```python
from build123d import *

# Parameters (mm, degrees)
F1_DEPTH = 11
F3_DEPTH = 25
F4_W     = 3.629314
F4_H     = 7.762888
F5_DEPTH = 35
F6_R     = 3
F7_DEPTH = 7.75
F8_R     = 1.5
F9_DEPTH = 25


with BuildPart() as f1:
    # F0 (on Top) → F1 (new body)
    with BuildSketch(Plane.XY):
        with BuildLine():
            Line((1.2, 0), (3, 0))
            ThreePointArc((3, 0), (2.12132, 2.12132), (0, 3))
            Line((0, 3), (0, 1.2))
            Line((0, 1.2), (1.2, 1.2))
            Line((1.2, 1.2), (1.2, 1.0315))
            Line((1.2, 1.0315), (1.2, 0.863))
            Line((1.2, 0.863), (1.2, 0))
        make_face()
        with BuildLine():
            ThreePointArc((0, -3), (2.12132, -2.12132), (3, 0))
            Line((3, 0), (1.2, 0))
            Line((1.2, 0), (1.2, -1.2))
            Line((1.2, -1.2), (0, -1.2))
            Line((0, -1.2), (0, -3))
        make_face()
        with BuildLine():
            Line((0, 1.2), (0, 3))
            ThreePointArc((0, 3), (-2.12132, 2.12132), (-3, 0))
            Line((-3, 0), (-1.2, 0))
            Line((-1.2, 0), (-1.2, 1.0315))
            Line((-1.2, 1.0315), (-1.2, 1.2))
            Line((-1.2, 1.2), (0, 1.2))
        make_face()
        with BuildLine():
            ThreePointArc((-3, 0), (-2.12132, -2.12132), (0, -3))
            Line((0, -3), (0, -1.2))
            Line((0, -1.2), (-1.2, -1.2))
            Line((-1.2, -1.2), (-1.2, 0))
            Line((-1.2, 0), (-3, 0))
        make_face()
    extrude(amount=F1_DEPTH)

    # F2 (on face) → F3 (cut)
    with BuildSketch(Plane.XY.offset(11)):
        with BuildLine():
            Line((1.814657, -2.388937), (-1.814657, -2.388937))
            ThreePointArc((-1.814657, -2.388937), (0, -3), (1.814657, -2.388937))
        make_face()
    extrude(amount=-F3_DEPTH, mode=Mode.SUBTRACT)

    # F4 (on face) → F5 (join)
    with BuildSketch(Plane.XZ.offset(2.388937)):
        with Locations((0, 3.881444)):
            Rectangle(F4_W, F4_H)
    extrude(amount=F5_DEPTH)

    # F6 (on face) → F7 (join)
    with BuildSketch(Plane.XY.offset(7.762888)):
        with Locations((0, -37.388937)):
            Circle(F6_R)
    extrude(amount=-F7_DEPTH)

    # F8 (on face) → F9 (cut)
    with BuildSketch(Plane.XY.offset(7.762888)):
        with Locations((0, -37.388937)):
            Circle(F8_R)
    extrude(amount=-F9_DEPTH, mode=Mode.SUBTRACT)


solid = f1.part
```
Source: CAD feature listing. Evaluate the final solid. Frame: model axes, mm. A direction names the side the tool comes from. Round coordinates to 2 decimals unless told otherwise and drop trailing zeros. Loops run counter-clockwise (first coordinate to the right, second up) from the corner with the lowest first, then second, coordinate; pieces in that order, holes last. Notation, with made-up numbers: M 60.25,1 L 65.25,1 A18 ccw 65.25,20 Z; hole C 54,-28.5 d6. An arc over 180 degrees is marked long. Use a Markdown table: item, result. Add a question column.
1. Line query: line 1 (Y direction, x = 1, z = 7); line 2 (Z direction, x = 1, y = -11); line 3 (X direction, y = -5, z = 1). Output: solid intervals per line, ascending.
2. Section query B-B on x = 0.5. Return the cut outline in (y, z).
3. Reachability of faces 4 (the flat face through (0, -21, 7.763)), 5 (the flat face through (1.2, 0, 5)), 6 (the flat face through (-1.4, 0.3, 11)) from +Z, -Z, +X, -X, +Y, -Y: full face, straight path, thin tool, end or side. Return the list, or none.
4. Mould query, pull axis Y, two halves, no side actions, for faces 1 (the flat face through (1.815, -16, 4)), 2 (the flat face through (0, -2.389, 9)), 3 (the flat face through (0, -17, 0)). Classes: pulls with the +Y half, pulls with the -Y half, needs draft (parallel to the pull), parting line crosses it, or undercut.
5. Section query A-A on z = 9.5. Return the cut outline in (x, y).
6. Section query D-D on y = -0.5. Return the cut outline in (x, z).
7. Section query C-C on z = 5. Give the number of separate pieces and of enclosed holes in the cut face, then the cut area to 3 significant figures.
8. Contact query for flat-ended pins moving along their axis: P1, Ø1, axis at x = -2, y = -24.5, coming from the +Z side; P2, Ø6, axis at y = -22.5, z = 3, coming from the -X side; P3, Ø0.7, axis at y = 0.5, z = 5.5, coming from the +X side; P4, Ø2, axis at y = -32.5, z = 9.5, coming from the +X side. Output: stop coordinate, or through.
Reported:
| question | item | result |
|---|---|---|
| 1 | line 1 | y = -40.22 to -38.51, -36.27 to -1.2, 1.2 to 2.83 |
| 1 | line 2 | z = 0 to 7.76 |
| 1 | line 3 | x = -1.81 to 1.81 |
| 2 | outline | M -40.35,0.01 L -38.8,0.01 L -38.8,7.76 L -40.35,7.76 Z; M -35.97,0 L -1.2,0 L -1.2,11 L -2.39,11 L -2.39,7.76 L -35.97,7.76 Z; M 1.2,0 L 2.96,0 L 2.96,11 L 1.2,11 Z |
| 3 | face 4 | +Z, +X, -X, -Y |
| 3 | face 5 | +Z, -Z |
| 3 | face 6 | +Z, +X, -X, +Y, -Y |
| 4 | face 1 | undercut |
| 4 | face 2 | pulls with the -Y half |
| 4 | face 3 | needs draft |
| 5 | outline | M -3,0 A3 ccw -1.81,-2.39 L 1.81,-2.39 A3 ccw 3,0 A3 ccw 0,3 A3 ccw Z; hole M -1.2,-1.2 L 1.2,-1.2 L 1.2,1.2 L -1.2,1.2 Z |
| 6 | outline | M -2.96,0 L -1.2,0 L -1.2,11 L -2.96,11 Z; M 1.2,0 L 2.96,0 L 2.96,11 L 1.2,11 Z |
| 7 | separate pieces | 1 |
| 7 | enclosed holes | 2 |
| 7 | area | 159 mm² |
| 8 | P1 | stops at z = 7.76 |
| 8 | P2 | stops at x = -1.81 |
| 8 | P3 | stops at x = 3 |
| 8 | P4 | passes through |
